```python
from build123d import *
from build123d import SkipClean  # not in build123d's __all__

# Parameters (mm, degrees)
F1_ANGLE = 340


with BuildPart() as f1:
    # F0 (on Front) → F1 (revolve)
    with BuildSketch(Plane.XZ):
        Polygon((-48.5273150222, 95.1958908392), (-51.4471201788, 83.3390055934), (71.3136761488, 50.8), (73.2494630124, 62.9177093663), align=None)
    revolve(axis=Axis((3.1582843512, 0, 0), (1, 0, 0)), revolution_arc=F1_ANGLE)

    # F2 (on face) → F3 (revolve)
    with BuildSketch(Plane(origin=(0, 0, 0), x_dir=(1, 0, 0), z_dir=(0, -0.9396926208, 0.3420201433))):
        Polygon((-7.8220407683, 84.4065412565), (-20.3833373413, 87.7360414852), (-25.218585377, 76.3868639802), (-13.9751803482, 73.4066843946), align=None)
    with SkipClean():  # cleaning this boolean's faces spoils the solid; the shape is the same uncleaned
        revolve(axis=Axis((73.2494630124, 0, 0), (-1, 0, 0)))


solid = f1.part
```
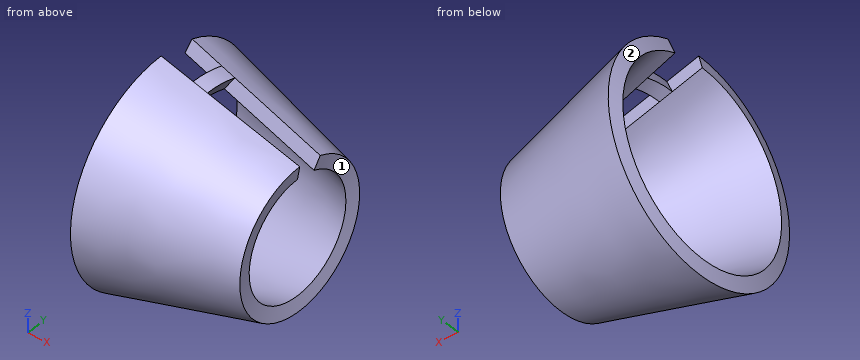
For this review, take the finished solid that the model builds, in its own axes (mm). Face numbers are marked on the shaded views. Coordinates: 2 decimals unless noted, no trailing zeros. Write each loop counter-clockwise with the first axis right and the second up, starting at its lowest first coordinate (ties: lowest second). Pieces come first, ordered by that corner, then holes.
(1) Add section B-B on x = -10.5. Give the boundary of the cut face in (y, z).
(2) Add section D-D on x = -42. Give the boundary of the cut face in (y, z).
(3) The part is to be moulded in two halves that separate along Y. For the marked faces 1 and 2, say which applies: +Y half, -Y half, draft (parallel to the pull), parting line (faces both ways), or undercut.
(4) For pin 1 Ø10 at (x, z) = (12, 63.5) entering from +Y; pin 2 Ø6 at (x, y) = (23, 19.5) entering from -Z; pin 3 Ø5 at (x, z) = (-35.5, 27.5) entering from -Y; pin 4 Ø12 at (y, z) = (34, -25.5) entering from +X (1 decimal), all flat-tipped, find the tip position at first contact; note any pin that passes through.
(5) Add section C-C on x = 54.5. Give the boundary of the cut face in (y, z).
(6) Add section A-A on z = 0. Give the boundary of the cut face in (x, y), then the cut area to 3 significant figures.
(7) Wall thickness on probe 1 along Y at (x, z) = (40.5, -3.5); probe 2 along Y at (x, z) = (31, 7); probe 3 along Z at (x, y) = (-8, -12): over which ranges is each line inside the solid? List them lowest first.
Answer sheet:
1. outline: circle Ø170.23 at (0, 0); hole (0, 72.49) arc R72.49 ccw (long way) to (24.79, 68.11) - (27.23, 74.82) arc R79.62 ccw to (0, 79.62) - close
2. outline: (0, 80.83) - (0, 93.47) arc R93.47 ccw (long way) to (31.97, 87.83) - (27.65, 75.96) arc R80.83 cw (long way) to start
3. face 1: undercut
3. face 2: parting line
4. pin 1: stops at y = 53.66
4. pin 2: stops at z = -74.81
4. pin 3: stops at y = -88.55
4. pin 4: passes through
5. outline: (0, 55.26) - (0, 67.89) arc R67.89 ccw (long way) to (23.22, 63.79) - (18.9, 51.92) arc R55.26 cw (long way) to start
6. outline: (-51.45, -83.34) - (-48.53, -95.2) - (73.25, -62.92) - (71.31, -50.8) - close; (-51.45, 83.34) - (71.31, 50.8) - (73.25, 62.92) - (-48.53, 95.2) - close
6. area: 3,090 mm2
7. probe 1: y = -71.51 to -58.86, 58.86 to 71.51
7. probe 2: y = -73.79 to -61.09, 61.09 to 73.79
7. probe 3: z = -83.6 to -70.81, 70.81 to 83.6
